Model file for the job. Use its own axes, mm. A direction names the side the tool comes from. Round coordinates to 2 decimals unless told otherwise and drop trailing zeros. Loops run counter-clockwise (first coordinate to the right, second up) from the corner with the lowest first, then second, coordinate; pieces in that order, holes last. Notation, with made-up numbers: (3.5, 72.5) -> (11.5, 72.5) arc R30 cw to (11.5, 99.5) -> close; hole circle Ø8 at (4, 0). An arc over 180 degrees is marked (long way). Use a Markdown table: item, result.
from build123d import *

# Parameters (mm, degrees)
SKETCH1_W               = 50.8
SKETCH1_H               = 25.4
SKETCH1_W_2             = 47.625
SKETCH1_H_2             = 22.225
BOSS_EXTRUDE1_DEPTH     = 180.975
SKETCH2_R               = 2.4892
CUT_EXTRUDE1_DEPTH      = 185.505475867
SKETCH9_W               = 31.75
SKETCH9_H               = 69.85
CUT_EXTRUDE2_DEPTH      = 23.8125
FILLET1_R               = 3.175
CUT_EXTRUDE3_DEPTH      = 184.189521057
CUT_EXTRUDE3_DEPTH_BACK = 184.189521057
SKETCH11_R              = 2.0193


with BuildPart() as part:
    # Sketch1 → Boss-Extrude1 (new body)
    with BuildSketch(Plane.XY):
        Rectangle(SKETCH1_W, SKETCH1_H)
        Rectangle(SKETCH1_W_2, SKETCH1_H_2, mode=Mode.SUBTRACT)
    extrude(amount=BOSS_EXTRUDE1_DEPTH)

    # Sketch2 → Cut-Extrude1 (cut, through all)
    with BuildSketch(Plane(origin=(0, 12.7, 0), x_dir=(1, 0, 0), z_dir=(0, 1, 0))):
        with Locations(Location((-12.7, -15.875, 0), (0, 0, 270))):
            Circle(SKETCH2_R)
        with Locations(Location((0, -15.875, 0), (0, 0, 270))):
            Circle(SKETCH2_R)
        with Locations(Location((12.7, -15.875, 0), (0, 0, 270))):
            Circle(SKETCH2_R)
        with Locations(Location((-12.7, -168.275, 0), (0, 0, 270))):
            Circle(SKETCH2_R)
        with Locations(Location((0, -168.275, 0), (0, 0, 270))):
            Circle(SKETCH2_R)
        with Locations(Location((12.7, -168.275, 0), (0, 0, 270))):
            Circle(SKETCH2_R)
        with Locations(Location((6.35, -33.3375, 0), (0, 0, 270))):
            Circle(SKETCH2_R)
        with Locations(Location((6.35, -46.0375, 0), (0, 0, 270))):
            Circle(SKETCH2_R)
    extrude(amount=-CUT_EXTRUDE1_DEPTH, mode=Mode.SUBTRACT)

    # Sketch9 → Cut-Extrude2 (cut)
    with BuildSketch(Plane(origin=(0, 12.7, 0), x_dir=(1, 0, 0), z_dir=(0, 1, 0))):
        with Locations((0, -98.425)):
            Rectangle(SKETCH9_W, SKETCH9_H)
    extrude(amount=-CUT_EXTRUDE2_DEPTH, mode=Mode.SUBTRACT)

    # Fillet1
    fillet1_edges = [part.edges().sort_by_distance(p)[0] for p in [
        (-15.875, 11.90625, 133.35),
        (-15.875, 11.90625, 63.5),
        (15.875, 11.90625, 63.5),
        (15.875, 11.90625, 133.35),
    ]]
    fillet(fillet1_edges, radius=FILLET1_R)

    # Sketch11 → Cut-Extrude3 (cut, two sides: drawn at the far end of the back side and taken through both)
    with BuildSketch(Plane(origin=(0, 0, 0), x_dir=(0, 0, -1), z_dir=(1, 0, 0)).offset(-CUT_EXTRUDE3_DEPTH_BACK)):
        with Locations((-130.175, 4.7625)):
            Circle(SKETCH11_R)
        with Locations((-130.175, -7.9375)):
            Circle(SKETCH11_R)
        with BuildLine():
            Line((-120.65, 7.9375), (-76.2, 7.9375))
            ThreePointArc((-76.2, 7.9375), (-73.025, 4.7625), (-76.2, 1.5875))
            Line((-76.2, 1.5875), (-120.65, 1.5875))
            ThreePointArc((-120.65, 1.5875), (-123.825, 4.7625), (-120.65, 7.9375))
        make_face()
    extrude(amount=CUT_EXTRUDE3_DEPTH + CUT_EXTRUDE3_DEPTH_BACK, mode=Mode.SUBTRACT)


solid = part.part
Q1. Band-saw the part on B-B, the plane x = 6.35. Give the number of separate pieces and of enclosed holes in the cut face, plus the area to 3 significant figures.
Results list:
| item | result |
|---|---|
| separate pieces | 7 |
| enclosed holes | 0 |
| area | 432 mm² |
Q2. Band-saw the part on C-C, the plane z = 38.5. Give the cut face in (x, y).
Results list:
| item | result |
|---|---|
| outline | (-25.4, -12.7) -> (25.4, -12.7) -> (25.4, 12.7) -> (-25.4, 12.7) -> close; hole (-23.81, -11.11) -> (23.81, -11.11) -> (23.81, 11.11) -> (-23.81, 11.11) -> close |
Q3. Pull direction Z, two halves, no side cores. Call faces 6 (the face through (0, -12.7, 89)), 7 (the face through (0, -12, 0)), 8 (the face through (-24.617, -7.849, 132.192)): released by +Z, released by -Z, zero draft, split by the parting line, or undercut.
Results list:
| item | result |
|---|---|
| face 6 | zero draft |
| face 7 | released by -Z |
| face 8 | undercut |
Q4. Band-saw the part on A-A, the plane y = -3.5. Give the cut face in (x, z) (1 decimal).
Results list:
| item | result |
|---|---|
| outline | (-25.4, 0) -> (-23.8, 0) -> (-23.8, 181) -> (-25.4, 181) -> close; (23.8, 0) -> (25.4, 0) -> (25.4, 181) -> (23.8, 181) -> close |
Q5. Drill centre lines: L1, parallel to Y at x = 14.5, z = 51.5; L2, parallel to X at y = 6.5, z = 43; L3, parallel to Y at x = -3.5, z = 116. Where is each one in solid material? Low to high. Write a range as from..to.
Results list:
| item | result |
|---|---|
| L1 | y = -12.7..-11.11, 11.11..12.7 |
| L2 | x = -25.4..-23.81, 23.81..25.4 |
| L3 | y = -12.7..-11.11 |
Q6. Flat gauge pins, fed straight in: pin 1 (3.5 mm diameter, centred on y = -7.94, z = 130.18, fed in from -X); pin 2 (8 mm diameter, centred on x = 0, z = 168.275, fed in from -Y); pin 3 (5 mm diameter, centred on x = 12.5, z = 124.5, fed in from +Y). Where does each tip first touch, or does it go through?
Results list:
| item | result |
|---|---|
| pin 1 | passes through |
| pin 2 | stops at y = -12.7 |
| pin 3 | stops at y = -11.11 |
Q7. Tool access for faces 1 (the face through (14.92, 11.895, 132.445)), 2 (the face through (25.4, 0, 89)), 3 (the face through (0, -11.112, 89)), 4 (the face through (0.11, -11.9, 13.39)), 5 (the face through (-24.617, 4.832, 73.026)): list every direction of +Z, -Z, +X, -X, +Y, -Y with a clear straight run to the whole face (end or side of a thin tool).
Results list:
| item | result |
|---|---|
| face 1 | +Y |
| face 2 | +Z, -Z, +X, +Y, -Y |
| face 3 | +Z, -Z |
| face 4 | +Y, -Y |
| face 5 | +X, -X |
